Check sheet for the modelled part. Datum: model origin and axes. Units: mm. A direction names the side the tool comes from. Round coordinates to 2 decimals unless told otherwise and drop trailing zeros. Write each loop counter-clockwise with the first axis right and the second up, starting at its lowest first coordinate (ties: lowest second). Pieces come first, ordered by that corner, then holes. Notation, with made-up numbers: M 58.5,10 L 107.5,10 A25 ccw 107.5,41 Z; hole C 63,-4 d3. An arc over 180 degrees is marked long. Answer in a Markdown table with one row per item.
```python
from build123d import *

# Parameters (mm, degrees)
F0_R     = 14.2875
F0_R_2   = 3.175
F1_DEPTH = 4.7625


# Not quite as in the source:
# - a feature names something its author has since deleted; it is built from what else it names


with BuildPart() as f1:
    # F0 (on Front) → F1 (new body)
    with BuildSketch(Plane.XZ):
        with BuildLine():
            Line((217.3001338382, 15.2277942336), (331.7059490892, 85.3303231618))
            Line((331.7059490892, 85.3303231618), (331.7059490892, 114.5403231618))
            ThreePointArc((331.7059490892, 114.5403231618), (329.8460771498, 119.0304512224), (325.3559490892, 120.8903231618))
            Line((325.3559490892, 120.8903231618), (0, 120.8903231618))
            Line((0, 120.8903231618), (-325.3559490892, 120.8903231618))
            ThreePointArc((-325.3559490892, 120.8903231618), (-329.8460771498, 119.0304512224), (-331.7059490892, 114.5403231618))
            Line((-331.7059490892, 114.5403231618), (-331.7059490892, 85.3303231618))
            Line((-331.7059490892, 85.3303231618), (-217.3001338382, 15.2277942336))
            ThreePointArc((-217.3001338382, 15.2277942336), (-199.5915875984, 11.4937311101), (-183.5057841229, 19.7872685874))
            Line((-183.5057841229, 19.7872685874), (-121.3841438293, 86.0923231618))
            Line((-121.3841438293, 86.0923231618), (0, 86.0923231618))
            Line((0, 86.0923231618), (121.3841438293, 86.0923231618))
            Line((121.3841438293, 86.0923231618), (183.5057841229, 19.7872685874))
            ThreePointArc((183.5057841229, 19.7872685874), (199.5915875984, 11.4937311101), (217.3001338382, 15.2277942336))
        make_face()
        with Locations((-203.2, 38.2389085481)):
            Circle(F0_R, mode=Mode.SUBTRACT)
        with Locations((203.2, 38.2389085481)):
            Circle(F0_R, mode=Mode.SUBTRACT)
        with Locations((-224.77598496, 112.7515938063)):
            Circle(F0_R_2, mode=Mode.SUBTRACT)
        with Locations((-173.97598496, 112.7515938063)):
            Circle(F0_R_2, mode=Mode.SUBTRACT)
        with Locations((-25.4, 112.7515938063)):
            Circle(F0_R_2, mode=Mode.SUBTRACT)
        with Locations((25.4, 112.7515938063)):
            Circle(F0_R_2, mode=Mode.SUBTRACT)
        with Locations((166.6059490892, 112.7515938063)):
            Circle(F0_R_2, mode=Mode.SUBTRACT)
        with Locations((217.4059490892, 112.7515938063)):
            Circle(F0_R_2, mode=Mode.SUBTRACT)
    extrude(amount=F1_DEPTH)


solid = f1.part
```
1. Access from +Z, -Z, +X, -X, +Y, -Y to the whole of each face (thin tool, end or side, straight path). Record for faces 1 (the face through (-190, -2.35, 32.77)), 2 (the face through (-152.88, -2.348, 52.476)).
Found:
| item | result |
|---|---|
| face 1 | +Y, -Y |
| face 2 | -Z, +Y, -Y |
2. Section check A-A, the plane x = -203.2. Record the cut outline in (y, z), and give its area (3 significant figures).
Found:
| item | result |
|---|---|
| outline | M -4.76,11.25 L 0,11.25 L 0,23.95 L -4.76,23.95 Z; M -4.76,52.53 L 0,52.53 L 0,120.89 L -4.76,120.89 Z |
| area | 386 mm2 |
3. Go/stop test with flat-tipped pins: pin 1 (1.4 mm diameter, centred on x = -53, y = -3.5, fed in from -Z); pin 2 (2 mm diameter, centred on y = -2, z = 24.5, fed in from -X). Record where each tip stops, or that it passes through.
Found:
| item | result |
|---|---|
| pin 1 | stops at z = 86.09 |
| pin 2 | stops at x = -234.06 |
4. Section check B-B, the plane z = 66.5. Record the cut outline in (x, y).
Found:
| item | result |
|---|---|
| outline | M -300.98,-4.76 L -139.74,-4.76 L -139.74,0 L -300.98,0 Z; M 139.74,-4.76 L 300.98,-4.76 L 300.98,0 L 139.74,0 Z |
5. Section check D-D, the plane x = -89. Record the cut outline in (y, z), and give its area (3 significant figures).
Found:
| item | result |
|---|---|
| outline | M -4.76,86.09 L 0,86.09 L 0,120.89 L -4.76,120.89 Z |
| area | 166 mm2 |
6. Scan lines: L1, parallel to X at y = -2.45, z = 49; L2, parallel to Z at x = 203.2, y = -2.85; L3, parallel to X at y = -0.7, z = 39.5. Record each from-to range of solid material in increasing order.
Found:
| item | result |
|---|---|
| L1 | x = -272.42 to -212.6, -193.8 to -156.14, 156.14 to 193.8, 212.6 to 272.42 |
| L2 | z = 11.25 to 23.95, 52.53 to 120.89 |
| L3 | x = -256.91 to -217.43, -188.97 to -165.04, 165.04 to 188.97, 217.43 to 256.91 |
7. Draft check along X on faces 3 (the face through (152.01, -2.348, 53.404)), 4 (the face through (-275.304, -2.348, 50.77)), 5 (the face through (273.702, -2.348, 49.788)), 6 (the face through (-5, 0, 91)). Enter one of: +X half, -X half, draft (parallel to the pull), parting line (faces both ways), or undercut.
Found:
| item | result |
|---|---|
| face 3 | undercut |
| face 4 | -X half |
| face 5 | +X half |
| face 6 | draft |
8. Section check C-C, the plane y = -2. Count the separate pieces of the cut face and the enclosed holes in it, and give its area (3 significant figures).
Found:
| item | result |
|---|---|
| separate pieces | 1 |
| enclosed holes | 8 |
| area | 38,800 mm2 |
